```python
from build123d import *

# Parameters (mm, degrees)
BASE_FLANGE1_DEPTH            = 1.21
M3_CLEARANCE_HOLE2_AT_2_COUNT = 2
M3_CLEARANCE_HOLE2_AT_2_PITCH = 66
M3_CLEARANCE_HOLE2_AT_3_COUNT = 2
M3_CLEARANCE_HOLE2_AT_3_PITCH = 86.678897774
FILLET1_R                     = 20
SKETCH62_W                    = 21.5
SKETCH62_H                    = 8.5
QRD_CLEARANCE_DEPTH           = 10
QRD_HOLES_D                   = 3.4
QRD_HOLES_DEPTH               = 1.27
QRD_HOLES_TIP                 = 1.021463052
M3_STEERING_BOX_D             = 3.4
M3_STEERING_BOX_DEPTH         = 3
M3_STEERING_BOX_TIP           = 1.021463052
EDGE_FLANGE1_STRIP_W          = 6.364
EDGE_FLANGE1_STRIP_H          = 1.21
EDGE_FLANGE1_STRIP_CUT_DEPTH  = 173
EDGE_FLANGE1_DEPTH            = 173
EDGE_FLANGE2_STRIP_W          = 6.364
EDGE_FLANGE2_STRIP_H          = 1.21
EDGE_FLANGE2_STRIP_CUT_DEPTH  = 140
EDGE_FLANGE2_DEPTH            = 140
EDGE_FLANGE3_STRIP_W          = 6.364
EDGE_FLANGE3_STRIP_H          = 1.21
EDGE_FLANGE3_STRIP_CUT_DEPTH  = 75
EDGE_FLANGE3_DEPTH            = 75
M3_CLEARANCE_HOLE3_D          = 3.4
M3_CLEARANCE_HOLE4_D          = 3.4
M3_CLEARANCE_HOLE5_D          = 3.4
M3_CLEARANCE_HOLE5_DEPTH      = 1.21
M3_CLEARANCE_HOLE6_D          = 3.4
M3_CLEARANCE_HOLE7_D          = 3.4
M3_CLEARANCE_HOLE7_DEPTH      = 1.21
M3_CLEARANCE_HOLE7_TIP        = 1.021463052
M3_CLEARANCE_HOLE8_D          = 3.4
M3_CLEARANCE_HOLE9_D          = 3.4
M3_CLEARANCE_HOLE10_D         = 3.4
M3_CLEARANCE_HOLE11_D         = 3.4


# Sheet-metal steps are written as plain solids
with BuildPart() as part:
    # Sketch1 → Base-Flange1 (new body)
    with BuildSketch(Plane(origin=(0, 0, 0), x_dir=(1, 0, 0), z_dir=(0, 1, 0))):
        Polygon((0, 0), (173, 0), (173, 100), (238, 100), (238, 175), (156.5, 175), (156.5, 300), (16.5, 300), (16.5, 175), (-65, 175), (-65, 100), (0, 100), align=None)
    extrude(amount=-BASE_FLANGE1_DEPTH)

    # Sketch28 → M3 Clearance Hole2 (revolve, cut)
    with BuildSketch(Plane(origin=(9.052, -1.21, -27.479586063), x_dir=(0, 0, -1), z_dir=(1, 0, 0))):
        Polygon((0, 0), (0, 2.291463052), (1.7, 1.27), (1.7, 0), align=None)
    m3_clearance_hole2 = revolve(axis=Axis((9.052, -7.56, -27.479586063), (0, 1, 0)), mode=Mode.SUBTRACT)

    # M3 Clearance Hole2 at 2: M3 Clearance Hole2 ×2
    with Locations(*[(i * M3_CLEARANCE_HOLE2_AT_2_PITCH, 0, 0) for i in range(1, M3_CLEARANCE_HOLE2_AT_2_COUNT)]):
        add(m3_clearance_hole2, mode=Mode.SUBTRACT)

    # M3 Clearance Hole2 at 3: M3 Clearance Hole2 ×2
    with Locations(*[Vector(0.38492784467456836, 0, -0.9229466693120418) * (i * M3_CLEARANCE_HOLE2_AT_3_PITCH) for i in range(1, M3_CLEARANCE_HOLE2_AT_3_COUNT)]):
        add(m3_clearance_hole2, mode=Mode.SUBTRACT)

    # Mirror3: M3 Clearance Hole2 across plane
    add(m3_clearance_hole2.mirror(Plane(origin=(86.5, 0, 0), x_dir=(0, 0, 1), z_dir=(1, 0, 0))), mode=Mode.SUBTRACT)

    # Mirror3 copy 1 sketch → Mirror3 copy 1 (revolve, cut)
    with BuildSketch(Plane(origin=(97.948, -1.21, -27.479586063), x_dir=(0, 0, -1), z_dir=(-1, 0, 0))):
        Polygon((0, 0), (0, -2.291463052), (1.7, -1.27), (1.7, 0), align=None)
    revolve(axis=Axis((97.948, -7.56, -27.479586063), (0, -1, 0)), mode=Mode.SUBTRACT)

    # Mirror3 copy 2 sketch → Mirror3 copy 2 (revolve, cut)
    with BuildSketch(Plane(origin=(130.582878701, -1.21, -107.479586063), x_dir=(0, 0, -1), z_dir=(-1, 0, 0))):
        Polygon((0, 0), (0, -2.291463052), (1.7, -1.27), (1.7, 0), align=None)
    revolve(axis=Axis((130.582878701, -7.56, -107.479586063), (0, -1, 0)), mode=Mode.SUBTRACT)

    # Fillet1
    fillet1_edges = [part.edges().sort_by_distance(p)[0] for p in [
        (0, -0.605, -100),
        (16.5, -0.605, -175),
        (156.5, -0.605, -175),
        (173, -0.605, -100),
    ]]
    fillet(fillet1_edges, radius=FILLET1_R)

    # Sketch62 → QRD Clearance (cut)
    with BuildSketch(Plane(origin=(0, 0, 0), x_dir=(1, 0, 0), z_dir=(0, 1, 0))):
        with Locations((86.5, 291.488)):
            Rectangle(SKETCH62_W, SKETCH62_H)
    extrude(amount=-QRD_CLEARANCE_DEPTH, mode=Mode.SUBTRACT)

    # QRD Holes
    with Locations(Plane(origin=(0, 0, 0), x_dir=(1, 0, 0), z_dir=(0, 1, 0))):
        with Locations((92, 280.488), (81, 280.488)):
            Hole(QRD_HOLES_D / 2, depth=QRD_HOLES_DEPTH)
            with Locations((0, 0, -(QRD_HOLES_DEPTH + QRD_HOLES_TIP / 2))):  # 118° drill point
                Cone(0, QRD_HOLES_D / 2, QRD_HOLES_TIP, mode=Mode.SUBTRACT)

    # M3 (Steering Box)
    with Locations(Plane(origin=(0, 0, 0), x_dir=(1, 0, 0), z_dir=(0, 1, 0))):
        with Locations((39.262, 262.238), (39.262, 207.762), (133.738, 207.762), (133.738, 262.238)):
            Hole(M3_STEERING_BOX_D / 2, depth=M3_STEERING_BOX_DEPTH)
            with Locations((0, 0, -(M3_STEERING_BOX_DEPTH + M3_STEERING_BOX_TIP / 2))):  # 118° drill point
                Cone(0, M3_STEERING_BOX_D / 2, M3_STEERING_BOX_TIP, mode=Mode.SUBTRACT)

    # Edge-Flange1 strip (across the edge) → Edge-Flange1 strip cut (cut)
    with BuildSketch(Plane(origin=(0, 0, 0), x_dir=(0, 0, -1), z_dir=(1, 0, 0))):
        with Locations((-1.21, -0.605)):
            Rectangle(EDGE_FLANGE1_STRIP_W, EDGE_FLANGE1_STRIP_H)
    extrude(amount=EDGE_FLANGE1_STRIP_CUT_DEPTH, mode=Mode.SUBTRACT)

    # Edge-Flange1 section (across the edge) → Edge-Flange1 (add)
    with BuildSketch(Plane(origin=(0, 0, 0), x_dir=(0, 0, -1), z_dir=(1, 0, 0))):
        with BuildLine():
            Line((0, 0.762), (0, 15))
            Line((0, 15), (1.21, 15))
            Line((1.21, 15), (1.21, 0.762))
            ThreePointArc((1.21, 0.762), (1.433184633, 0.223184633), (1.972, 0))
            Line((1.972, 0), (1.972, -1.21))
            ThreePointArc((1.972, -1.21), (0.577585428, -0.632414572), (0, 0.762))
        make_face()
    extrude(amount=EDGE_FLANGE1_DEPTH)

    # Edge-Flange2 strip (across the edge) → Edge-Flange2 strip cut (cut)
    with BuildSketch(Plane(origin=(156.5, 0, -300), x_dir=(0, 0, 1), z_dir=(-1, 0, 0))):
        with Locations((-1.21, -0.605)):
            Rectangle(EDGE_FLANGE2_STRIP_W, EDGE_FLANGE2_STRIP_H)
    extrude(amount=EDGE_FLANGE2_STRIP_CUT_DEPTH, mode=Mode.SUBTRACT)

    # Edge-Flange2 section (across the edge) → Edge-Flange2 (add)
    with BuildSketch(Plane(origin=(156.5, 0, -300), x_dir=(0, 0, 1), z_dir=(-1, 0, 0))):
        with BuildLine():
            Line((0, 0.762), (0, 15))
            Line((0, 15), (1.21, 15))
            Line((1.21, 15), (1.21, 0.762))
            ThreePointArc((1.21, 0.762), (1.433184633, 0.223184633), (1.972, 0))
            Line((1.972, 0), (1.972, -1.21))
            ThreePointArc((1.972, -1.21), (0.577585428, -0.632414572), (0, 0.762))
        make_face()
    extrude(amount=EDGE_FLANGE2_DEPTH)

    # Edge-Flange3 strip (across the edge) → Edge-Flange3 strip cut (cut)
    with BuildSketch(Plane(origin=(238, 0, -100), x_dir=(-1, 0, 0), z_dir=(0, 0, -1))):
        with Locations((-1.21, -0.605)):
            Rectangle(EDGE_FLANGE3_STRIP_W, EDGE_FLANGE3_STRIP_H)
    edge_flange3_strip_cut = extrude(amount=EDGE_FLANGE3_STRIP_CUT_DEPTH, mode=Mode.SUBTRACT)

    # Edge-Flange3 section (across the edge) → Edge-Flange3 (add)
    with BuildSketch(Plane(origin=(238, 0, -100), x_dir=(-1, 0, 0), z_dir=(0, 0, -1))):
        with BuildLine():
            Line((0, 0.762), (0, 15))
            Line((0, 15), (1.21, 15))
            Line((1.21, 15), (1.21, 0.762))
            ThreePointArc((1.21, 0.762), (1.433184633, 0.223184633), (1.972, 0))
            Line((1.972, 0), (1.972, -1.21))
            ThreePointArc((1.972, -1.21), (0.577585428, -0.632414572), (0, 0.762))
        make_face()
    edge_flange3 = extrude(amount=EDGE_FLANGE3_DEPTH)

    # Mirror4: Edge-Flange3 strip cut, Edge-Flange3 across plane
    add(edge_flange3_strip_cut.mirror(Plane(origin=(86.5, 0, 0), x_dir=(0, 0, 1), z_dir=(1, 0, 0))), mode=Mode.SUBTRACT)
    add(edge_flange3.mirror(Plane(origin=(86.5, 0, 0), x_dir=(0, 0, 1), z_dir=(1, 0, 0))))

    # M3 Clearance Hole3 (through all)
    with Locations(Plane(origin=(50.766060613, 0, -139.899791502), x_dir=(1, 0, 0), z_dir=(0, 1, 0))):
        with Locations((-28.266060613, 124.338208498), (-28.266060613, 94.338208498)):
            Hole(M3_CLEARANCE_HOLE3_D / 2)

    # M3 Clearance Hole4 (through all)
    with Locations(Plane(origin=(50.766060613, 0, -139.899791502), x_dir=(1, 0, 0), z_dir=(0, 1, 0))):
        with Locations((99.733939387, 124.338208498), (99.733939387, 94.338208498)):
            Hole(M3_CLEARANCE_HOLE4_D / 2)

    # M3 Clearance Hole5
    with Locations(Plane.XY):
        with Locations((86.5, 7.881)):
            Hole(M3_CLEARANCE_HOLE5_D / 2, depth=M3_CLEARANCE_HOLE5_DEPTH)

    # M3 Clearance Hole6 (through all)
    with Locations(Plane(origin=(238, 0, 0), x_dir=(0, 0, -1), z_dir=(1, 0, 0))):
        with Locations((137.5, 7.881)):
            Hole(M3_CLEARANCE_HOLE6_D / 2)

    # M3 Clearance Hole7
    with Locations(Plane(origin=(0, 0, -300), x_dir=(-1, 0, 0), z_dir=(0, 0, -1))):
        with Locations((-86.5, 7.881)):
            Hole(M3_CLEARANCE_HOLE7_D / 2, depth=M3_CLEARANCE_HOLE7_DEPTH)
            with Locations((0, 0, -(M3_CLEARANCE_HOLE7_DEPTH + M3_CLEARANCE_HOLE7_TIP / 2))):  # 118° drill point
                Cone(0, M3_CLEARANCE_HOLE7_D / 2, M3_CLEARANCE_HOLE7_TIP, mode=Mode.SUBTRACT)

    # M3 Clearance Hole8 (through all)
    with Locations(Plane(origin=(50.766060613, 0, -139.899791502), x_dir=(1, 0, 0), z_dir=(0, 1, 0))):
        with Locations((-25.095060613, 146.719208498), (96.562939387, 146.719208498)):
            Hole(M3_CLEARANCE_HOLE8_D / 2)

    # M3 Clearance Hole9 (through all)
    with Locations(Plane(origin=(50.766060613, 0, -139.899791502), x_dir=(1, 0, 0), z_dir=(0, 1, 0))):
        with Locations((-102.385060613, -30.728791502), (-102.385060613, 25.929208498)):
            Hole(M3_CLEARANCE_HOLE9_D / 2)

    # M3 Clearance Hole10 (through all)
    with Locations(Plane(origin=(50.766060613, 0, -139.899791502), x_dir=(1, 0, 0), z_dir=(0, 1, 0))):
        with Locations((173.852939387, 25.929208498), (173.852939387, -30.728791502)):
            Hole(M3_CLEARANCE_HOLE10_D / 2)

    # M3 Clearance Hole11 (through all)
    with Locations(Plane(origin=(50.766060613, 0, -139.899791502), x_dir=(1, 0, 0), z_dir=(0, 1, 0))):
        with Locations((113.062939387, -129.018791502), (-41.595060613, -129.018791502)):
            Hole(M3_CLEARANCE_HOLE11_D / 2)


solid = part.part
```
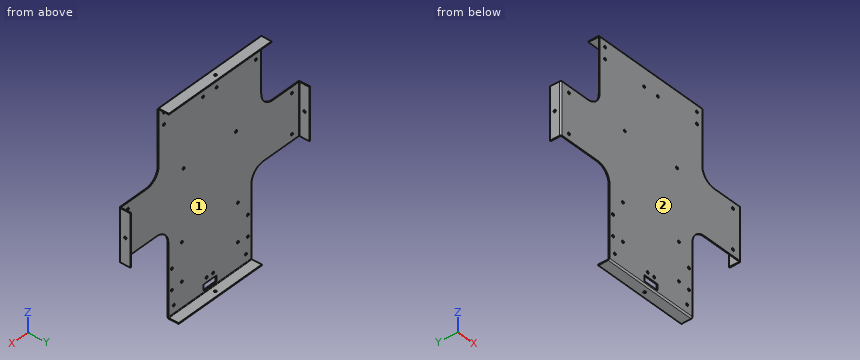
Geometry: final body of the model. Coordinates: model frame, mm. Face numbers are marked on the shaded views. Round coordinates to 2 decimals unless told otherwise and drop trailing zeros. Write each loop counter-clockwise with the first axis right and the second up, starting at its lowest first coordinate (ties: lowest second). Pieces come first, ordered by that corner, then holes. Notation, with made-up numbers: (32.25, 43) -> (41.25, 43) arc R21 ccw to (41.25, 73) -> close; hole circle Ø11 at (-5, -22). An arc over 180 degrees is marked (long way). Use CSV: the item, a comma, the result in double quotes. Start each with the question number.
Q1. Pull-direction query (X, two-part tool) for the marked faces 1 and 2; classes: pulls with the +X half, pulls with the -X half, needs draft (parallel to the pull), parting line crosses it, or undercut.
Q2. First-contact query: pin 1 Ø2.5 at (x, z) = (133.738, -262.238) entering from -Y; pin 2 Ø3 at (x, z) = (23, -160.5) entering from +Y. Flat tips, straight axial feed; report the tip coordinate or a pass-through.
Q3. Line query: L1, parallel to Z at x = 72.5, y = 4; L2, parallel to Z at x = 22.5, y = -0.65; L3, parallel to Z at x = 22.5, y = -0.85. Output: solid intervals per line, ascending.
Q4. Section A-A (z = -245). Return loops of the section in (x, y), plus the area to 3 significant figures.
Q5. Section B-B (x = -9). Return loops of the section in (y, z), plus the area to 3 significant figures.
Result sheet:
1,face 1,"undercut"
1,face 2,"needs draft"
2,pin 1,"through"
2,pin 2,"y = 0"
3,L1,"-300 to -298.79, -1.21 to 0"
3,L2,"-299.4 to -265.94, -262.54 to -235.94, -232.54 to -0.6"
3,L3,"-299.16 to -265.94, -262.54 to -235.94, -232.54 to -0.84"
4,outline,"(16.5, -1.21) -> (156.5, -1.21) -> (156.5, 0) -> (16.5, 0) -> close"
4,area,"169 mm²"
5,outline,"(-1.21, -175) -> (0, -175) -> (0, -96.7) -> (-1.21, -96.7) -> close"
5,area,"94.7 mm²"
